from build123d import *

# Parameters (mm, degrees)
SKETCH1_W           = 76.76
SKETCH1_H           = 75
BOSS_EXTRUDE1_DEPTH = 6.35
SKETCH2_R           = 6.815
CUT_EXTRUDE1_DEPTH  = 55.033294366
SKETCH3_R           = 1.8
CUT_EXTRUDE2_DEPTH  = 55.033294366
CHAMFER1_SIZE       = 3.58


with BuildPart() as part:
    # Sketch1 → Boss-Extrude1 (new body)
    with BuildSketch(Plane(origin=(0, 0, 0), x_dir=(1, 0, 0), z_dir=(0, 1, 0))):
        Rectangle(SKETCH1_W, SKETCH1_H)
    extrude(amount=BOSS_EXTRUDE1_DEPTH)

    # Sketch2 → Cut-Extrude1 (cut, through all)
    with BuildSketch(Plane(origin=(0, 6.35, 0), x_dir=(1, 0, 0), z_dir=(0, 1, 0))):
        with Locations(Location((0, 0, 0), (0, 0, 270))):
            Circle(SKETCH2_R)
    extrude(amount=-CUT_EXTRUDE1_DEPTH, mode=Mode.SUBTRACT)

    # Sketch3 → Cut-Extrude2 (cut, through all)
    with BuildSketch(Plane(origin=(0, 6.35, 0), x_dir=(1, 0, 0), z_dir=(0, 1, 0))):
        with Locations(Location((-30.97, 30.09, 0), (0, 0, 270))):
            Circle(SKETCH3_R)
        with Locations(Location((-30.97, -30.09, 0), (0, 0, 270))):
            Circle(SKETCH3_R)
        with Locations(Location((30.97, -30.09, 0), (0, 0, 270))):
            Circle(SKETCH3_R)
        with Locations(Location((30.97, 30.09, 0), (0, 0, 270))):
            Circle(SKETCH3_R)
        with Locations(Location((-30.97, 0, 0), (0, 0, 270))):
            Circle(SKETCH3_R)
        with Locations(Location((30.97, 0, 0), (0, 0, 270))):
            Circle(SKETCH3_R)
    extrude(amount=-CUT_EXTRUDE2_DEPTH, mode=Mode.SUBTRACT)

    # Chamfer1
    chamfer1_edges = [part.edges().sort_by_distance(p)[0] for p in [
        (0, 0, -6.815),
    ]]
    chamfer(chamfer1_edges, length=CHAMFER1_SIZE)


solid = part.part
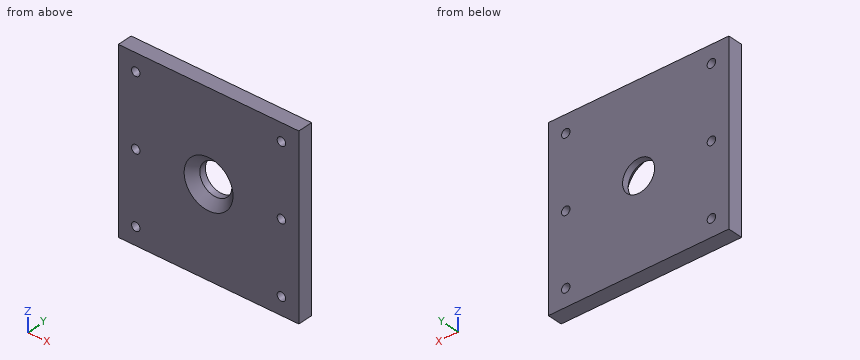
Work out the finished part from the listing and answer in its coordinate system (mm). Round coordinates to 2 decimals unless told otherwise and drop trailing zeros. Write each loop counter-clockwise with the first axis right and the second up, starting at its lowest first coordinate (ties: lowest second). Pieces come first, ordered by that corner, then holes.
1) A cutting plane is placed at B-B (x = -30.97). Give the vertices of the cut face in (y, z), plus the area to 3 significant figures.
2) Straight lines are drawn through the part: line 1 (X direction, y = 3.5, z = 30.09); line 2 (X direction, y = 3, z = -29.5); line 3 (X direction, y = 3.25, z = 0) (3 decimals). For each, find the intervals that lie inside material, in ascending order.
3) A cutting plane is placed at C-C (z = -30.09). Give the vertices of the cut face in (x, y), plus the area to 3 significant figures.
4) A cutting plane is placed at D-D (x = 0). Give the vertices of the cut face in (y, z) (3 decimals).
5) Given pin 1 Ø4.5 at (x, z) = (30.97, -30.09) entering from +Y; pin 2 Ø2 at (x, z) = (30.97, 0) entering from -Y; pin 3 Ø5 at (x, z) = (3, -6.5) entering from -Y, each flat-ended and moving along its own axis, determine where each tip first touches the part or whether it passes through.
6) A cutting plane is placed at A-A (z = 0). Give the vertices of the cut face in (x, y) (3 decimals).
Completed:
1. outline: (0, -37.5) - (6.35, -37.5) - (6.35, -31.89) - (0, -31.89) - close; (0, -28.29) - (6.35, -28.29) - (6.35, -1.8) - (0, -1.8) - close; (0, 1.8) - (6.35, 1.8) - (6.35, 28.29) - (0, 28.29) - close; (0, 31.89) - (6.35, 31.89) - (6.35, 37.5) - (0, 37.5) - close
1. area: 408 mm2
2. line 1: x = -38.38 to -32.77, -29.17 to 29.17, 32.77 to 38.38
2. line 2: x = -38.38 to -32.67, -29.27 to 29.27, 32.67 to 38.38
2. line 3: x = -38.38 to -32.77, -29.17 to -7.145, 7.145 to 29.17, 32.77 to 38.38
3. outline: (-38.38, 0) - (-32.77, 0) - (-32.77, 6.35) - (-38.38, 6.35) - close; (-29.17, 0) - (29.17, 0) - (29.17, 6.35) - (-29.17, 6.35) - close; (32.77, 0) - (38.38, 0) - (38.38, 6.35) - (32.77, 6.35) - close
3. area: 442 mm2
4. outline: (0, -37.5) - (6.35, -37.5) - (6.35, -6.815) - (3.58, -6.815) - (0, -10.395) - close; (0, 10.395) - (3.58, 6.815) - (6.35, 6.815) - (6.35, 37.5) - (0, 37.5) - close
5. pin 1: stops at y = 6.35
5. pin 2: passes through
5. pin 3: stops at y = 0.74
6. outline: (-38.38, 0) - (-32.77, 0) - (-32.77, 6.35) - (-38.38, 6.35) - close; (-29.17, 0) - (-10.395, 0) - (-6.815, 3.58) - (-6.815, 6.35) - (-29.17, 6.35) - close; (6.815, 3.58) - (10.395, 0) - (29.17, 0) - (29.17, 6.35) - (6.815, 6.35) - close; (32.77, 0) - (38.38, 0) - (38.38, 6.35) - (32.77, 6.35) - close
